Design review of the part built by this model. Coordinates are the model's own, in mm. Coordinates: 2 decimals unless noted, no trailing zeros. Write each loop counter-clockwise with the first axis right and the second up, starting at its lowest first coordinate (ties: lowest second). Pieces come first, ordered by that corner, then holes.
Q1. Take a section at B-B, the plane z = 4. State how many separate pieces and enclosed holes the cut face has, plus the area to 3 significant figures.
Q2. For L1, parallel to X at y = 65.5, z = 2.5; L2, parallel to X at y = -11, z = 5.75, list the stretches that pass through material, from the lowest coordinate up.
Q3. Take a section at A-A, the plane y = -38.1. Write out the cut boundary in (x, z) (3 decimals), plus the area to 3 significant figures.
Q4. The part is to be moulded in two halves that separate along Y. For faces 1 (the cylindrical face through (-13.11, 28.55, 3.13)), 2 (the flat face through (-25.4, -1, 3)), 3 (the flat face through (0, -101.6, 3)), say which applies: released by +Y, released by -Y, zero draft, split by the parting line, or undercut.
from build123d import *

# Parameters (mm, degrees)
SKETCH1_W           = 50.8
SKETCH1_H           = 203.2
SKETCH1_R           = 3.175
BOSS_EXTRUDE1_DEPTH = 6.35


with BuildPart() as part:
    # Sketch1 → Boss-Extrude1 (new body)
    with BuildSketch(Plane.XY):
        Rectangle(SKETCH1_W, SKETCH1_H)
        with Locations((-12.7, 88.9)):
            Circle(SKETCH1_R, mode=Mode.SUBTRACT)
        with Locations((12.7, 88.9)):
            Circle(SKETCH1_R, mode=Mode.SUBTRACT)
        with Locations((12.7, 76.2)):
            Circle(SKETCH1_R, mode=Mode.SUBTRACT)
        with Locations((12.7, 63.5)):
            Circle(SKETCH1_R, mode=Mode.SUBTRACT)
        with Locations((12.7, 50.8)):
            Circle(SKETCH1_R, mode=Mode.SUBTRACT)
        with Locations((12.7, 38.1)):
            Circle(SKETCH1_R, mode=Mode.SUBTRACT)
        with Locations((12.7, 25.4)):
            Circle(SKETCH1_R, mode=Mode.SUBTRACT)
        with Locations((12.7, 12.7)):
            Circle(SKETCH1_R, mode=Mode.SUBTRACT)
        with Locations((12.7, 0)):
            Circle(SKETCH1_R, mode=Mode.SUBTRACT)
        with Locations((12.7, -12.7)):
            Circle(SKETCH1_R, mode=Mode.SUBTRACT)
        with Locations((12.7, -25.4)):
            Circle(SKETCH1_R, mode=Mode.SUBTRACT)
        with Locations((12.7, -38.1)):
            Circle(SKETCH1_R, mode=Mode.SUBTRACT)
        with Locations((-12.7, -50.8)):
            Circle(SKETCH1_R, mode=Mode.SUBTRACT)
        with Locations((12.7, -50.8)):
            Circle(SKETCH1_R, mode=Mode.SUBTRACT)
        with Locations((-12.7, -63.5)):
            Circle(SKETCH1_R, mode=Mode.SUBTRACT)
        with Locations((12.7, -63.5)):
            Circle(SKETCH1_R, mode=Mode.SUBTRACT)
        with Locations((-12.7, -76.2)):
            Circle(SKETCH1_R, mode=Mode.SUBTRACT)
        with Locations((12.7, -76.2)):
            Circle(SKETCH1_R, mode=Mode.SUBTRACT)
        with Locations((-12.7, -88.9)):
            Circle(SKETCH1_R, mode=Mode.SUBTRACT)
        with Locations((12.7, -88.9)):
            Circle(SKETCH1_R, mode=Mode.SUBTRACT)
        with Locations((-12.7, 76.2)):
            Circle(SKETCH1_R, mode=Mode.SUBTRACT)
        with Locations((-12.7, 63.5)):
            Circle(SKETCH1_R, mode=Mode.SUBTRACT)
        with Locations((-12.7, 50.8)):
            Circle(SKETCH1_R, mode=Mode.SUBTRACT)
        with Locations((-12.7, 38.1)):
            Circle(SKETCH1_R, mode=Mode.SUBTRACT)
        with Locations((-12.7, 25.4)):
            Circle(SKETCH1_R, mode=Mode.SUBTRACT)
        with Locations((-12.7, 12.7)):
            Circle(SKETCH1_R, mode=Mode.SUBTRACT)
        with Locations((-12.7, 0)):
            Circle(SKETCH1_R, mode=Mode.SUBTRACT)
        with Locations((-12.7, -12.7)):
            Circle(SKETCH1_R, mode=Mode.SUBTRACT)
        with Locations((-12.7, -25.4)):
            Circle(SKETCH1_R, mode=Mode.SUBTRACT)
        with Locations((-12.7, -38.1)):
            Circle(SKETCH1_R, mode=Mode.SUBTRACT)
    extrude(amount=BOSS_EXTRUDE1_DEPTH)


solid = part.part
Responses:
1. separate pieces: 1
1. enclosed holes: 30
1. area: 9,370 mm2
2. L1: x = -25.4 to -15.17, -10.23 to 10.23, 15.17 to 25.4
2. L2: x = -25.4 to -15.38, -10.02 to 10.02, 15.38 to 25.4
3. outline: (-25.4, 0) - (-15.875, 0) - (-15.875, 6.35) - (-25.4, 6.35) - close; (-9.525, 0) - (9.525, 0) - (9.525, 6.35) - (-9.525, 6.35) - close; (15.875, 0) - (25.4, 0) - (25.4, 6.35) - (15.875, 6.35) - close
3. area: 242 mm2
4. face 1: undercut
4. face 2: zero draft
4. face 3: released by -Y
